Part model, mm, in its own coordinate system. Face numbers are marked on the shaded views. A direction names the side the tool comes from. Coordinates: 2 decimals unless noted, no trailing zeros. Loops run counter-clockwise (first coordinate to the right, second up) from the corner with the lowest first, then second, coordinate; pieces in that order, holes last. Notation, with made-up numbers: M 58,63.25 L 85,63.25 A32 cw 85,94.25 Z; hole C 56,86 d4. An arc over 180 degrees is marked long. Answer as a JSON object with one key per item and string values. Group by question number.
1. Saw through at A-A on x = 41.5. Write the cut outline in (y, z).
2. 3-axis set-ups, long thin cutter, end or side, ignore diameter. For the marked faces 1 and 2: which of +Z, -Z, +X, -X, +Y, -Y reach the whole face in a straight line?
3. Drill centre lines: L1, parallel to Y at x = -18, z = 14.25; L2, parallel to Y at x = -34, z = 12.5; L3, parallel to X at y = -28.5, z = 11. Where is each one in solid material? Low to high.
4. Saw through at B-B on y = -24. Write the cut outline in (x, z), then the cut area to 3 significant figures.
5. Mould opens along X. For the marked faces 3, 4, 5 and 6 say: released by +X, released by -X, zero draft, split by the parting line, or undercut.
6. Saw through at C-C on z = 11.5. Write the cut outline in (x, y).
7. Drop a flat-ended pin along its axis: pin 1 Ø3 at (x, y) = (-8, -9.5) entering from -Z. Give the stop position or say it passes through.
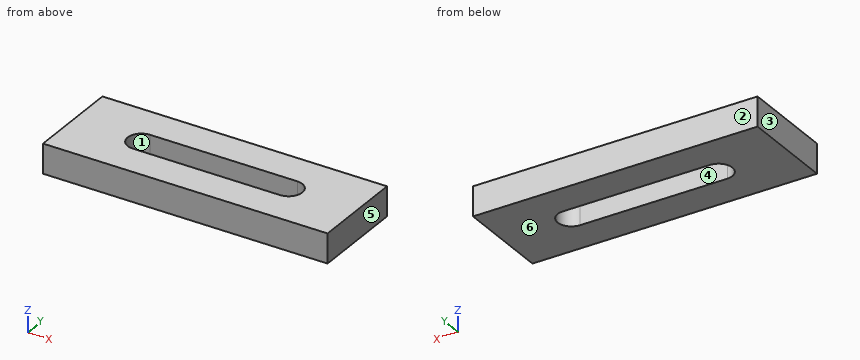
from build123d import *

# Parameters (mm, degrees)
F0_W     = 145
F0_H     = 48
F1_DEPTH = 15
F2_W     = 145
F2_H     = 12
F3_DEPTH = 15


with BuildPart() as f1:
    # F0 (on Top) → F1 (new body)
    with BuildSketch(Plane.XY):
        with Locations((9.905382, -24)):
            Rectangle(F0_W, F0_H)
        with BuildLine():
            ThreePointArc((-27.594618, -31), (-34.594618, -24), (-27.594618, -17))
            Line((-27.594618, -17), (47.405382, -17))
            ThreePointArc((47.405382, -17), (54.405382, -24), (47.405382, -31))
            Line((47.405382, -31), (-27.594618, -31))
        make_face(mode=Mode.SUBTRACT)
    extrude(amount=F1_DEPTH)

    # F2 (on Top) → F3 (join)
    with BuildSketch(Plane.XY):
        with Locations((9.905382, -6)):
            Rectangle(F2_W, F2_H)
    extrude(amount=F3_DEPTH)


solid = f1.part
Outcome:
{
 "1": {"outline": "M -48,0 L -31,0 L -31,15 L -48,15 Z; M -17,0 L 0,0 L 0,15 L -17,15 Z"},
 "2": {"face 1": "+Z, -Z", "face 2": "+Z, -Z, +X, -X, +Y"},
 "3": {"L1": "y = -48 to -31, -17 to 0", "L2": "y = -48 to -26.82, -21.18 to 0", "L3": "x = -62.59 to -32.96, 52.77 to 82.41"},
 "4": {"outline": "M -62.59,0 L -34.59,0 L -34.59,15 L -62.59,15 Z; M 54.41,0 L 82.41,0 L 82.41,15 L 54.41,15 Z", "area": "840 mm²"},
 "5": {"face 3": "released by -X", "face 4": "undercut", "face 5": "released by +X", "face 6": "zero draft"},
 "6": {"outline": "M -62.59,-48 L 82.41,-48 L 82.41,0 L -62.59,0 Z; hole M -27.59,-31 L 47.41,-31 A7 ccw 47.41,-17 L -27.59,-17 A7 ccw Z"},
 "7": {"pin 1": "stops at z = 0"}
}
